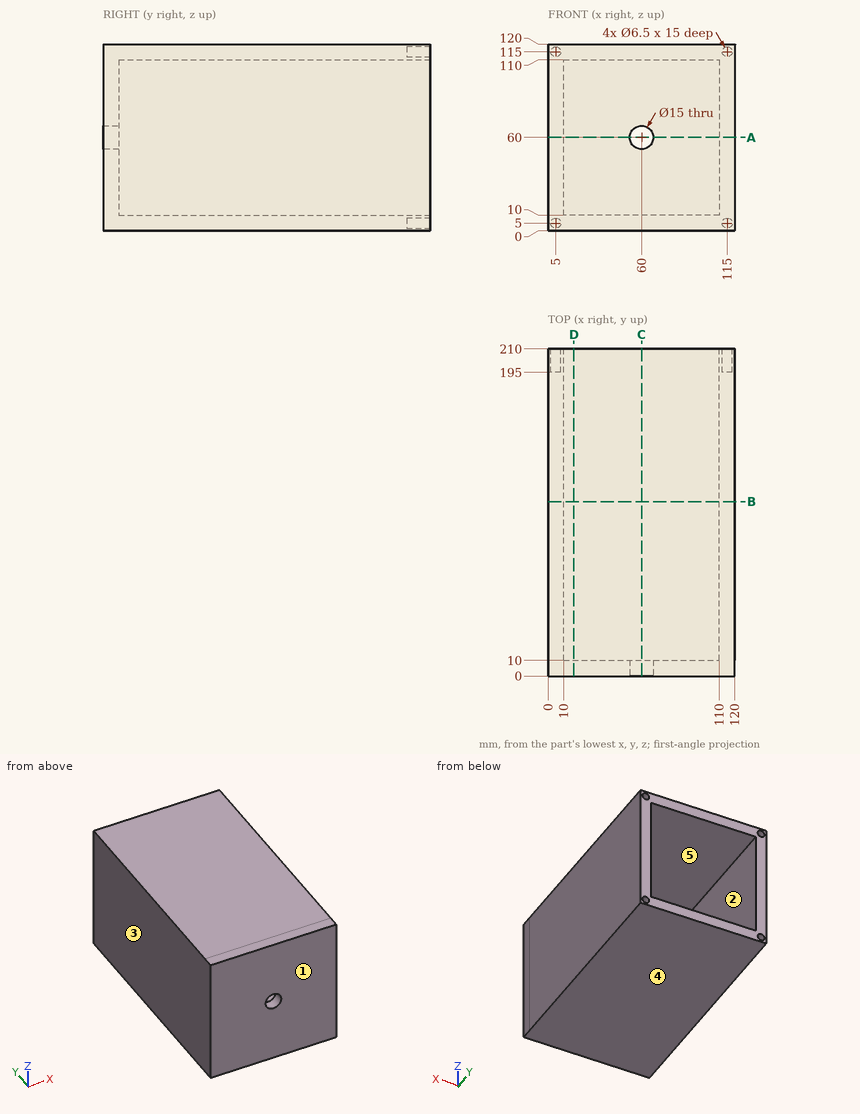
Drawing for the job (mm, zero at the part's lowest x, y, z). A direction names the side the tool comes from. Coordinates: 2 decimals unless noted, no trailing zeros. Loops run counter-clockwise (first coordinate to the right, second up) from the corner with the lowest first, then second, coordinate; pieces in that order, holes last. Notation, with made-up numbers: (-2.75, 61.25) - (13.25, 61.25) arc R19 cw to (13.25, 74.25) - close; hole circle Ø3 at (60, 33). An arc over 180 degrees is marked (long way). Return JSON: item names as keys, results as strings.
1. Band-saw the part on B-B (y = 112). Give the cut face in (x, z).
Result:
{"outline": "(0, 0) - (120, 0) - (120, 120) - (0, 120) - close; hole (10, 10) - (110, 10) - (110, 110) - (10, 110) - close"}
2. Band-saw the part on C-C (x = 60). Give the cut face in (y, z).
Result:
{"outline": "(0, 0) - (210, 0) - (210, 10) - (10, 10) - (10, 52.5) - (0, 52.5) - close; (0, 67.5) - (10, 67.5) - (10, 110) - (210, 110) - (210, 120) - (0, 120) - close"}
3. Band-saw the part on A-A (z = 60). Give the cut face in (x, y), and give its area (3 significant figures).
Result:
{"outline": "(0, 0) - (52.5, 0) - (52.5, 10) - (10, 10) - (10, 210) - (0, 210) - close; (67.5, 0) - (120, 0) - (120, 210) - (110, 210) - (110, 10) - (67.5, 10) - close", "area": "5,050 mm2"}
4. Probe L1, parallel to X at y = 128.5, z = 55.5; L2, parallel to Y at x = 76, z = 17. List the from-to ranges inside material, lowest first. Write a range as from..to.
Result:
{"L1": "x = 0..10, 110..120", "L2": "y = 0..10"}
5. Drop flat-ended pins along their axis: pin 1 (13.5 mm diameter, centred on x = 60, z = 60, fed in from +Y); pin 2 (2 mm diameter, centred on x = 3.5, z = 6.5, fed in from +Y). Give the stop position or say it passes through.
Result:
{"pin 1": "passes through", "pin 2": "stops at y = 195"}
6. 3-axis set-ups, long thin cutter, end or side, ignore diameter. For the marked faces 4 and 5: which of +Z, -Z, +X, -X, +Y, -Y reach the whole face in a straight line?
Result:
{"face 4": "-Z, +X, -X, +Y, -Y", "face 5": "+Y"}
7. Mould opens along X. For the marked faces 1, 2 and 3 say: released by +X, released by -X, zero draft, split by the parting line, or undercut.
Result:
{"face 1": "zero draft", "face 2": "undercut", "face 3": "released by -X"}
8. Band-saw the part on D-D (x = 16.5). Give the cut face in (y, z), and give its area (3 significant figures).
Result:
{"outline": "(0, 0) - (210, 0) - (210, 10) - (10, 10) - (10, 110) - (210, 110) - (210, 120) - (0, 120) - close", "area": "5,200 mm2"}
